Part model, mm, in its own coordinate system. A direction names the side the tool comes from. Round coordinates to 2 decimals unless told otherwise and drop trailing zeros. Write each loop counter-clockwise with the first axis right and the second up, starting at its lowest first coordinate (ties: lowest second). Pieces come first, ordered by that corner, then holes.
```python
from build123d import *

# Parameters (mm, degrees)
MODEL_R             = 4.911595
BOSS_EXTRUDE1_DEPTH = 10


with BuildPart() as part:
    # Model → Boss-Extrude1 (new body)
    with BuildSketch(Plane.XY):
        Polygon((109.372327, 95.103157), (110.762604, 95.280824), (111.808486, 95.159378), (114.324954, 94.041578), (114.324954, 92.475166), (111.808486, 91.357365), (110.762604, 91.235919), (109.372327, 91.413587), (108.74316, 88.657038), (110.072845, 88.213892), (110.96246, 87.650678), (112.744724, 85.551724), (112.065082, 84.140432), (109.312829, 84.225186), (108.317826, 84.569557), (107.142317, 85.332849), (105.379438, 83.122268), (106.385168, 82.146081), (106.942314, 81.252653), (107.637374, 78.588263), (106.412702, 77.611622), (103.96978, 78.882138), (103.222733, 79.62412), (102.494814, 80.821857), (99.94738, 79.59508), (100.42996, 78.279193), (100.544289, 77.232507), (100.014481, 74.530399), (98.48734, 74.18184), (96.837602, 76.386481), (96.486466, 77.379116), (96.350314, 78.774073), (93.522876, 78.774073), (93.386724, 77.379116), (93.035588, 76.386481), (91.38585, 74.18184), (89.858709, 74.530399), (89.328902, 77.232507), (89.44323, 78.279193), (89.92581, 79.59508), (87.378376, 80.821857), (86.650457, 79.62412), (85.90341, 78.882138), (83.460488, 77.611622), (82.235816, 78.588263), (82.930876, 81.252653), (83.488022, 82.146081), (84.493752, 83.122268), (82.730873, 85.332849), (81.555364, 84.569557), (80.560362, 84.225186), (77.808108, 84.140432), (77.128466, 85.551724), (78.91073, 87.650678), (79.800346, 88.213892), (81.13003, 88.657038), (80.500863, 91.413587), (79.110586, 91.235919), (78.064704, 91.357365), (75.548236, 92.475166), (75.548236, 94.041578), (78.064704, 95.159378), (79.110586, 95.280824), (80.500863, 95.103157), (81.13003, 97.859706), (79.800346, 98.302851), (78.91073, 98.866065), (77.128466, 100.96502), (77.808108, 102.376311), (80.560362, 102.291557), (81.555364, 101.947187), (82.730873, 101.183894), (84.493752, 103.394476), (83.488022, 104.370663), (82.930876, 105.264091), (82.235816, 107.928481), (83.460488, 108.905122), (85.90341, 107.634605), (86.650457, 106.892623), (87.378376, 105.694886), (89.92581, 106.921664), (89.44323, 108.237551), (89.328902, 109.284237), (89.858709, 111.986345), (91.38585, 112.334904), (93.035588, 110.130263), (93.386724, 109.137628), (93.522876, 107.742671), (96.350314, 107.742671), (96.486466, 109.137628), (96.837602, 110.130263), (98.48734, 112.334904), (100.014481, 111.986345), (100.544289, 109.284237), (100.42996, 108.237551), (99.94738, 106.921664), (102.494814, 105.694886), (103.222733, 106.892623), (103.96978, 107.634605), (106.412702, 108.905122), (107.637374, 107.928481), (106.942314, 105.264091), (106.385168, 104.370663), (105.379438, 103.394476), (107.142317, 101.183894), (108.317826, 101.947187), (109.312829, 102.291557), (112.065082, 102.376311), (112.744724, 100.96502), (110.96246, 98.866065), (110.072845, 98.302851), (108.74316, 97.859706), align=None)
        with Locations((94.936589262, 93.258379)):
            Circle(MODEL_R, mode=Mode.SUBTRACT)
    extrude(amount=BOSS_EXTRUDE1_DEPTH)


solid = part.part
```
Q1. Which spindle directions (+Z, -Z, +X, -X, +Y, -Y) get a long thin tool onto all of the face, cutting with end or side? Do faces 1 (the flat face through (79.36, 98.58, 4.93)), 2 (the flat face through (109.4, 88.44, 4.93)), 3 (the flat face through (88.634, 106.3, 4.93)), 4 (the flat face through (93.21, 109.64, 4.93)). Say none if no direction does.
Values follow:
face 1: +Z, -Z, -X
face 2: +Z, -Z, +X
face 3: +Z, -Z
face 4: +Z, -Z, +Y
Q2. Cut at B-B on y = 89.5. Write the cut outline in (x, z).
Values follow:
outline: (80.94, 0) - (91.77, 0) - (91.77, 10) - (80.94, 10) - close; (98.1, 0) - (108.94, 0) - (108.94, 10) - (98.1, 10) - close
Q3. Drop flat-ended pins along their axis: pin 1 (10 mm diameter, centred on x = 109, y = 86.5, fed in from -Z); pin 2 (1.5 mm diameter, centred on y = 91, z = 3, fed in from -X); pin 3 (2 mm diameter, centred on x = 95, z = 8, fed in from +Y); pin 4 (5 mm diameter, centred on x = 95, z = 4, fed in from +Y). Give the stop position or say it passes through.
Values follow:
pin 1: stops at z = 0
pin 2: stops at x = 77.18
pin 3: stops at y = 107.74
pin 4: stops at y = 111.02
Q4. Cut at A-A on x = 95. Write the cut outline in (y, z).
Values follow:
outline: (78.77, 0) - (88.35, 0) - (88.35, 10) - (78.77, 10) - close; (98.17, 0) - (107.74, 0) - (107.74, 10) - (98.17, 10) - close
Q5. Mould opens along Y. For faces 5 (the flat face through (101.2, 80.2, 4.9)), 6 (the flat face through (90.633, 74.354, 4.93)), 7 (the flat face through (107.02, 108.42, 4.93)) say: +Y half, -Y half, draft (parallel to the pull), parting line (faces both ways), or undercut.
Values follow:
face 5: undercut
face 6: -Y half
face 7: +Y half
Q6. Wall check: L1, parallel to Y at x = 95, z = 7; L2, parallel to X at y = 85, z = 4; L3, parallel to Y at x = 78.5, z = 8.75 (3 decimals). Give the ranges that are in metal, low to high.
Values follow:
L1: y = 78.77 to 88.35, 98.17 to 107.74
L2: x = 77.39 to 82.22, 83 to 106.88, 107.65 to 112.48
L3: y = 84.162 to 87.167, 91.307 to 95.21, 99.35 to 102.355
Q7. Cut at C-C on y = 99.5. Write the cut outline in (x, z).
Values follow:
outline: (78.37, 0) - (111.5, 0) - (111.5, 10) - (78.37, 10) - close
